Input: dimensioned drawing with shaded views. Units: mm. Origin: part minimum x, y, z. A direction names the side the tool comes from. Round coordinates to 2 decimals unless told otherwise and drop trailing zeros. Loops run counter-clockwise (first coordinate to the right, second up) from the corner with the lowest first, then second, coordinate; pieces in that order, holes last. Notation, with made-up numbers: M -30.75,6 L -2.75,6 A20 cw -2.75,18 Z; hole C -33,64 d7. An arc over 180 degrees is marked long. Put each result on its own line as item: value. Start each with the question number.
1) Reachability of the marked faces 1, 2 and 3 from +Z, -Z, +X, -X, +Y, -Y: full face, straight path, thin tool, end or side. Return the list, or none.
2) Line query: probe 1 along Z at (x, y) = (16.5, 2.75); probe 2 along Z at (x, y) = (8.75, 6); probe 3 along Y at (x, z) = (10, 5). Output: solid intervals per line, ascending.
3) Section C-C on z = 17. Output: boundary loops of the cut face in (x, y).
4) Section B-B on x = 10. Output: boundary loops of the cut face in (y, z), plus the area to 3 significant figures.
5) Section D-D on z = 30.5. Output: boundary loops of the cut face in (x, y), plus the area to 3 significant figures.
6) Section A-A on y = 10. Output: boundary loops of the cut face in (x, z).
7) Pin query (flat end, axial travel): pin 1 (5 mm diameter, centred on x = 5, y = 16, fed in from +Z); pin 2 (4 mm diameter, centred on x = 10, y = 6.5, fed in from -Z); pin 3 (5 mm diameter, centred on x = 9, y = 4, fed in from +Z); pin 4 (5 mm diameter, centred on y = 2, z = 11.5, fed in from +X). Return the tip coordinate at first contact, or that it passes through.
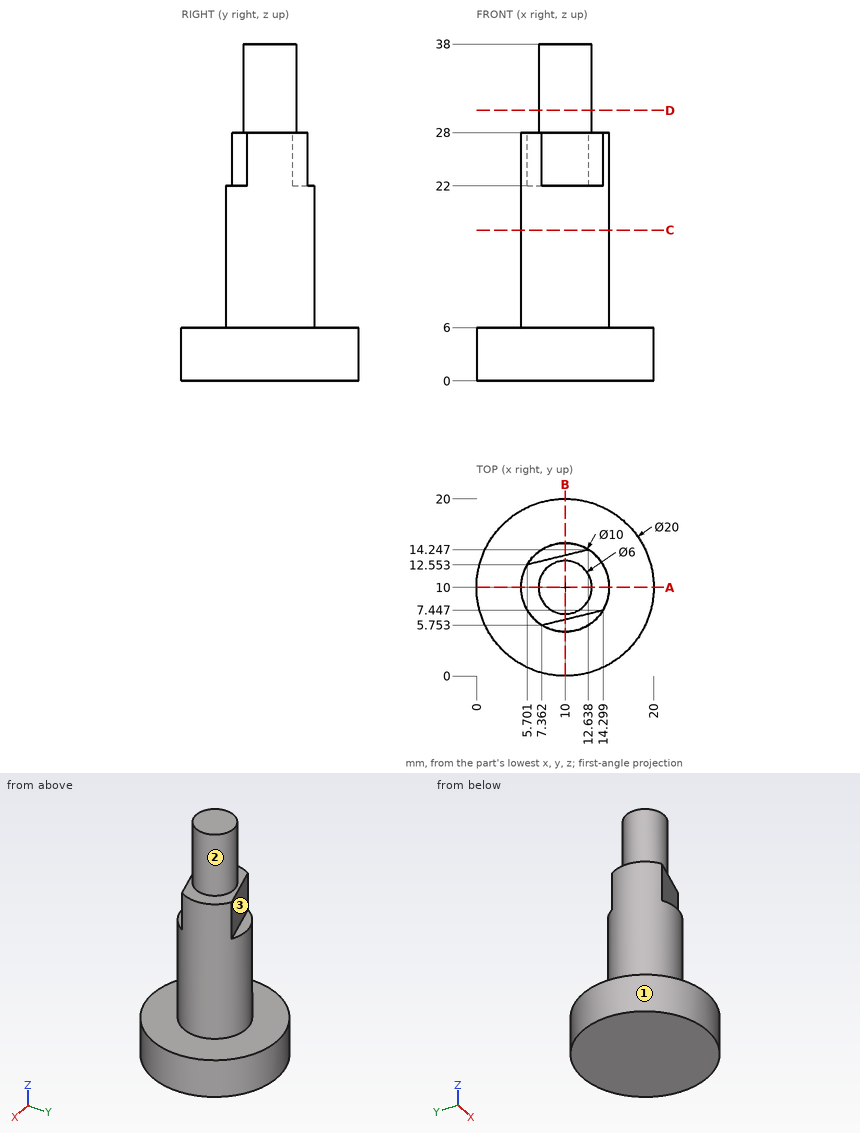
Geometry results:
1. face 1: +Z, -Z
1. face 2: +Z
1. face 3: +Z, -X, +Y
2. probe 1: z = 0 to 6
2. probe 2: z = 0 to 22
2. probe 3: y = 0 to 20
3. outline: C 10,10 d10
4. outline: M 0,0 L 20,0 L 20,6 L 15,6 L 15,22 L 13.6,22 L 13.6,28 L 13,28 L 13,38 L 7,38 L 7,28 L 6.4,28 L 6.4,22 L 5,22 L 5,6 L 0,6 Z
4. area: 383 mm²
5. outline: C 10,10 d6
5. area: 28.3 mm²
6. outline: M 0,0 L 20,0 L 20,6 L 15,6 L 15,28 L 13,28 L 13,38 L 7,38 L 7,28 L 5,28 L 5,6 L 0,6 Z
7. pin 1: stops at z = 6
7. pin 2: stops at z = 0
7. pin 3: stops at z = 28
7. pin 4: passes through
